```python
from build123d import *

# Parameters (mm, degrees)
F2_W     = 21.976557381
F2_H     = 31.7907221615
F3_DEPTH = 22.225
F1_W     = 15.621
F1_H     = 15.875
F1_H_2   = 0.635
F4_DEPTH = 28.6157221615
F5_DEPTH = 7.62


with BuildPart() as f3:
    # F2 (on Top) → F3 (new body)
    with BuildSketch(Plane.XY):
        with Locations((-0.0027786905, 15.8953610808)):
            Rectangle(F2_W, F2_H)
    extrude(amount=F3_DEPTH)

    # F1 (on Front) → F4 (cut, through all)
    with BuildSketch(Plane.XZ):
        with Locations((0, 11.1125)):
            Rectangle(F1_W, F1_H)
        with Locations((0, 2.8575)):
            Rectangle(F1_W, F1_H_2)
    extrude(amount=-F4_DEPTH, mode=Mode.SUBTRACT)

    # F1 (on Front) → F5 (join)
    with BuildSketch(Plane.XZ):
        with Locations((0, 2.8575)):
            Rectangle(F1_W, F1_H_2)
    extrude(amount=-F5_DEPTH)


solid = f3.part
```
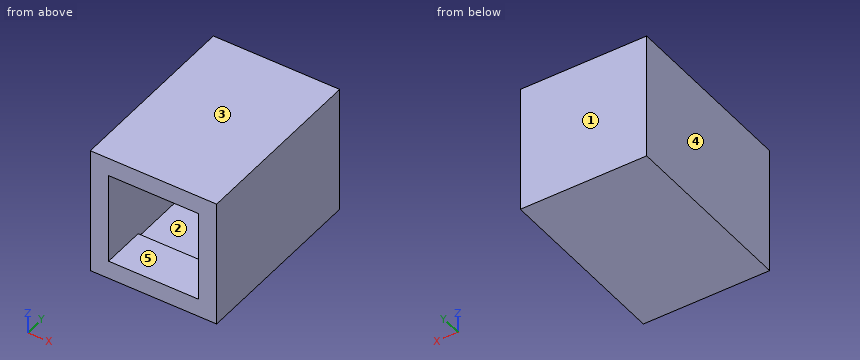
Build history of the part. All positions in model axes, mm. Face numbers are marked on the shaded views. A direction names the side the tool comes from. Round coordinates to 2 decimals unless told otherwise and drop trailing zeros. Order: outer loops, then holes, each group sorted by start corner. A loop starts at its lowest first (then second) coordinate and runs counter-clockwise, first axis right, second up. Notation, with made-up numbers: (51, 0) -> (81, 0) arc R29 ccw to (81, 35) -> close; hole circle Ø5 at (84.25, 7.5). An arc over 180 degrees is marked (long way). Answer in a Markdown table with one row per item.
1) Pin check, flat tip, straight feed: P1, Ø4.5, axis at x = 1.5, z = 13, coming from the -Y side. Stop position of the tip, or through.
Values:
| item | result |
|---|---|
| P1 | y = 28.62 |
2) Band-saw the part on C-C on z = 10.25. Give the cut face in (x, y), and give its area (3 significant figures).
Values:
| item | result |
|---|---|
| outline | (-10.99, 0) -> (-7.81, 0) -> (-7.81, 28.62) -> (7.81, 28.62) -> (7.81, 0) -> (10.99, 0) -> (10.99, 31.79) -> (-10.99, 31.79) -> close |
| area | 252 mm2 |
3) Which spindle directions (+Z, -Z, +X, -X, +Y, -Y) get a long thin tool onto all of the face, cutting with end or side? Do the marked faces 4 and 5. Say none if no direction does.
Values:
| item | result |
|---|---|
| face 4 | +Z, -Z, -X, +Y, -Y |
| face 5 | -Y |
4) Band-saw the part on B-B on x = 3.75. Give the cut face in (y, z) (3 decimals).
Values:
| item | result |
|---|---|
| outline | (0, 0) -> (31.791, 0) -> (31.791, 22.225) -> (0, 22.225) -> (0, 19.05) -> (28.616, 19.05) -> (28.616, 2.54) -> (7.62, 2.54) -> (7.62, 3.175) -> (0, 3.175) -> close |
5) Mould opens along Y. For the marked faces 1, 2 and 3 say: released by +Y, released by -Y, zero draft, split by the parting line, or undercut.
Values:
| item | result |
|---|---|
| face 1 | released by +Y |
| face 2 | undercut |
| face 3 | zero draft |
6) Wall check: L1, parallel to X at y = 28.5, z = 9.25; L2, parallel to Z at x = 5.25, y = 6 (3 decimals); L3, parallel to Z at x = 4.75, y = 8 (3 decimals). Give the ranges that are in metal, low to high.
Values:
| item | result |
|---|---|
| L1 | -10.99 to -7.81, 7.81 to 10.99 |
| L2 | 0 to 3.175, 19.05 to 22.225 |
| L3 | 0 to 2.54, 19.05 to 22.225 |
